Model file for the job. Use its own axes, mm. A direction names the side the tool comes from. Round coordinates to 2 decimals unless told otherwise and drop trailing zeros. Loops run counter-clockwise (first coordinate to the right, second up) from the corner with the lowest first, then second, coordinate; pieces in that order, holes last. Notation, with made-up numbers: M 73,21.25 L 115,21.25 A14 cw 115,28.25 Z; hole C -4.5,-22 d10. An arc over 180 degrees is marked long. Use a Markdown table: item, result. Add a question column.
Q1. Tool access for faces 1 (the face through (-304.8, 56, -75)), 2 (the face through (-128.937, 287.419, -85.928)), 3 (the face through (-128.173, -3.131, -83.829)): list every direction of +Z, -Z, +X, -X, +Y, -Y with a clear straight run to the whole face (end or side of a thin tool).
Q2. Cut at D-D (z = -76.2). Give the cut face in (x, y) (3 decimals).
Q3. Cut at C-C (y = 432). Give the cut face in (x, z), plus the area to 3 significant figures.
Q4. Probe line 1 (Y direction, x = -157.5, z = -30); line 2 (X direction, y = 235.5, z = -78.5); line 3 (X direction, y = 154, z = -97). List the from-to ranges inside material, lowest first. Write a range as from..to.
Q5. Cut at A-A (x = -152.4). Give the cut face in (y, z) (3 decimals).
Q6. Cut at B-B (z = -41). Give the cut face in (x, y).
Q7. Pin check, flat tips, straight feed: pin 1 (4 mm diameter, centred on x = -45.5, z = -85, fed in from -Y); pin 2 (8 mm diameter, centred on x = -146, z = -102, fed in from -Y). Stop position of each tip, or through.
Autodesk Inventor part; units mm, degrees
ref_plane "YZ Plane" through (0, 0, 0) normal (1, 0, 0) x (0, 1, 0)
ref_plane "XZ Plane" through (0, 0, 0) normal (0, 1, 0) x (-1, 0, 0)
ref_plane "XY Plane" through (0, 0, 0) normal (0, 0, 1) x (1, 0, 0)
sketch "Sketch1" plane through (0, 0, 0) normal (0, 1, 0) x (-1, 0, 0)
  line L0 (0, 0) -> (304.8, 0)
  line L1 (304.8, 0) -> (304.8, -152.4)
  line L2 (304.8, -152.4) -> (0, -152.4)
  line L3 (0, -152.4) -> (0, 0)
  dimension "d0" = 304.8
  dimension "d1" = 152.4
extrude "Extrusion1" add sketch "Sketch1" along normal blind 114.3
sketch "Sketch2" plane through (0, 114.3, 0) normal (0, 1, 0) x (1, 0, 0)
  circle A0 centre (-152.4, 76.2) radius 25.4
  line L0 (0, 0) -> (0, 152.4)
  line L1 (0, 152.4) -> (-304.8, 152.4)
  dimension "d4" = 152.4
  dimension "d5" = 76.2
  dimension "d6" = 50.8
extrude "Extrusion2" add sketch "Sketch2" along normal blind 355.6
sketch "Sketch3" plane through (0, 0, 0) normal (1, 0, 0) x (0, 0, -1)
  line L0 (152.4, 0) -> (152.4, 114.3)
  line L1 (0, 0) -> (152.4, 0)
  line L2 (152.4, 0) -> (152.4, 114.3)
  line L3 (152.4, 114.3) -> (0, 114.3)
  line L4 (0, 114.3) -> (0, 0)
chamfer "Chamfer1" distance 6.35 angle 45 1 edges at (0, 114.3, -76.2)
chamfer "Chamfer2" distance 6.35 angle 45 1 edges at (0, 53.975, 0)
chamfer "Chamfer3" distance 6.35 angle 45 1 edges at (0, 0, -79.375)
chamfer "Chamfer4" distance 6.35 angle 45 1 edges at (0, 57.15, -152.4)
chamfer "Chamfer5" distance 6.35 angle 45 4 edges at (-304.8, 114.3, -76.2) (-304.8, 57.15, -152.4) (-304.8, 57.15, 0) (-304.8, 0, -76.2)
chamfer "Chamfer6" distance 4.445 angle 45 1 edges at (-177.8, 469.9, -76.2)
sketch "Sketch4" plane through (0, 0, 0) normal (0, -1, 0) x (1, 0, 0)
  circle A0 centre (-152.4, -76.2) radius 25.4
  circle A1 centre (-152.4, -76.2) radius 25.4
  point P0 (0, 0)
extrude "Extrusion3" add sketch "Sketch4" along normal blind 6.35
properties part number "Mjolnir"
Checked values:
| question | item | result |
|---|---|---|
| 1 | face 1 | +Z, -Z, -X, +Y, -Y |
| 1 | face 2 | +Y |
| 1 | face 3 | -Y |
| 2 | outline | M -304.8,6.35 L -298.45,0 L -177.8,0 L -177.8,-6.35 L -127,-6.35 L -127,0 L -6.35,0 L 0,6.35 L 0,107.95 L -6.35,114.3 L -127,114.3 L -127,465.455 L -131.445,469.9 L -173.355,469.9 L -177.8,465.455 L -177.8,114.3 L -298.45,114.3 L -304.8,107.95 Z |
| 3 | outline | C -152.4,-76.2 d50.8 |
| 3 | area | 2,030 mm^2 |
| 4 | line 1 | y = 0..114.3 |
| 4 | line 2 | x = -177.7..-127.1 |
| 4 | line 3 | x = -166.98..-137.82 |
| 5 | outline | M -6.35,-101.6 L 0,-101.6 L 0,-152.4 L 114.3,-152.4 L 114.3,-101.6 L 465.455,-101.6 L 469.9,-97.155 L 469.9,-55.245 L 465.455,-50.8 L 114.3,-50.8 L 114.3,0 L 0,0 L 0,-50.8 L -6.35,-50.8 Z |
| 6 | outline | M -304.8,6.35 L -298.45,0 L -6.35,0 L 0,6.35 L 0,107.95 L -6.35,114.3 L -298.45,114.3 L -304.8,107.95 Z |
| 7 | pin 1 | stops at y = 0 |
| 7 | pin 2 | stops at y = -6.35 |
